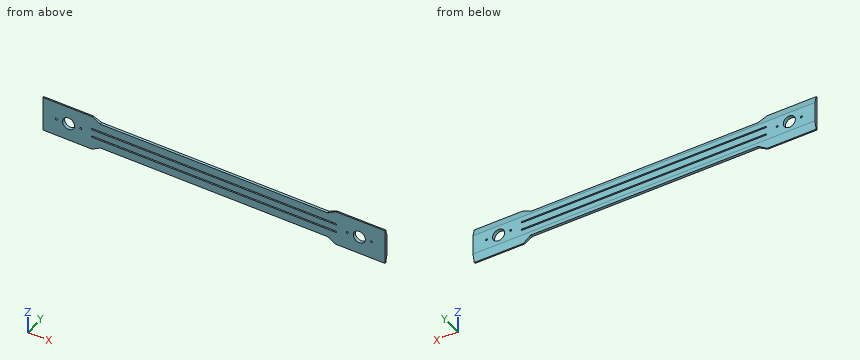
from build123d import *

# Parameters (mm, degrees)
EXTRUDE_1_DEPTH     = 25
SKETCH_2_R          = 45
SKETCH_2_R_2        = 7
CUT_EXTRUDE_1_DEPTH = 1277.880965478
CUT_EXTRUDE_2_DEPTH = 1277.880965478
CUT_EXTRUDE_3_DEPTH = 2544.447463582


with BuildPart() as part:
    # 草图1 → 凸台-拉伸1 (new body)
    with BuildSketch(Plane(origin=(0, 0, 0), x_dir=(1, 0, 0), z_dir=(0, 1, 0))):
        Polygon((-1270, 130), (-1270, -130), (-905, -130), (-844.378221735, -95), (844.378221735, -95), (905, -130), (1270, -130), (1270, 130), (905, 130), (844.378221735, 95), (-844.378221735, 95), (-905, 130), align=None)
    extrude(amount=EXTRUDE_1_DEPTH)

    # 草图2 → 切除-拉伸1 (cut, through all)
    with BuildSketch(Plane(origin=(0, 25, 0), x_dir=(1, 0, 0), z_dir=(0, 1, 0))):
        with Locations(Location((-1080, 0, 0), (0, 0, 270))):
            Circle(SKETCH_2_R)
        with Locations(Location((-1170, 0, 0), (0, 0, 270))):
            Circle(SKETCH_2_R_2)
        with Locations(Location((-990, 0, 0), (0, 0, 270))):
            Circle(SKETCH_2_R_2)
    cut_extrude_1 = extrude(amount=-CUT_EXTRUDE_1_DEPTH, mode=Mode.SUBTRACT)

    # 镜向1: 切除-拉伸1 across plane
    add(cut_extrude_1.mirror(Plane(origin=(0, 0, 0), x_dir=(0, 0, 1), z_dir=(1, 0, 0))), mode=Mode.SUBTRACT)

    # 草图3 → 切除-拉伸2 (cut, through all)
    with BuildSketch(Plane(origin=(0, 25, 0), x_dir=(1, 0, 0), z_dir=(0, 1, 0))):
        with BuildLine():
            Line((-905, -35), (905, -35))
            ThreePointArc((905, -35), (910, -30), (905, -25))
            Line((905, -25), (-905, -25))
            ThreePointArc((-905, -25), (-910, -30), (-905, -35))
        make_face()
    cut_extrude_2 = extrude(amount=-CUT_EXTRUDE_2_DEPTH, mode=Mode.SUBTRACT)

    # 镜向2: 切除-拉伸2 across plane
    add(cut_extrude_2.mirror(Plane.XY), mode=Mode.SUBTRACT)

    # 草图6 → 切除-拉伸3 (cut, through all)
    with BuildSketch(Plane(origin=(1270, 0, 0), x_dir=(0, 0, -1), z_dir=(1, 0, 0))):
        Polygon((-73, 25), (-130, 10), (-130, 25), align=None)
        Polygon((73, 25), (130, 10), (130, 25), align=None)
    extrude(amount=-CUT_EXTRUDE_3_DEPTH, mode=Mode.SUBTRACT)


solid = part.part
Geometry: final body of the model. Coordinates: model frame, mm. Coordinates: 2 decimals unless noted, no trailing zeros. Loops run counter-clockwise (first coordinate to the right, second up) from the corner with the lowest first, then second, coordinate; pieces in that order, holes last. Notation, with made-up numbers: (-38.75, 27) - (-13.75, 27) arc R14 ccw to (-13.75, 37) - close; hole circle Ø4 at (5, 11.5). An arc over 180 degrees is marked (long way). Put each result on its own line as item: value. Start each with the question number.
Q1. Cut plane B-B, the plane x = -712.5. Return loops of the section in (y, z).
Q2. Pin query (flat end, axial travel): pin 1 Ø3 at (x, z) = (402, -15) entering from -Y; pin 2 Ø7.5 at (x, y) = (-176.5, 7.5) entering from -Z; pin 3 Ø1 at (x, y) = (616.5, 17) entering from +Z. Return the tip coordinate at first contact, or that it passes through.
Q3. Cut plane A-A, the plane x = 1080. Return loops of the section in (y, z).
Q4. Line query: line 1 (Z direction, x = -444.5, y = 13.5); line 2 (Z direction, x = 1170, y = 9.5); line 3 (Z direction, x = -848.5, y = 5). Output: solid intervals per line, ascending.
Filled sheet:
1. outline: (0, -95) - (19.21, -95) - (25, -73) - (25, -35) - (0, -35) - close; (0, -25) - (25, -25) - (25, 25) - (0, 25) - close; (0, 35) - (25, 35) - (25, 73) - (19.21, 95) - (0, 95) - close
2. pin 1: y = 0
2. pin 2: z = -95
2. pin 3: z = 95
3. outline: (0, -130) - (10, -130) - (25, -73) - (25, -45) - (0, -45) - close; (0, 45) - (25, 45) - (25, 73) - (10, 130) - (0, 130) - close
4. line 1: -95 to -35, -25 to 25, 35 to 95
4. line 2: -130 to -7, 7 to 130
4. line 3: -97.38 to -35, -25 to 25, 35 to 97.38
